Model file for the job. Use its own axes, mm. A direction names the side the tool comes from. Give positions to 0.01 mm unless a question says otherwise; leave off trailing zeros. Order: outer loops, then holes, each group sorted by start corner. A loop starts at its lowest first (then second) coordinate and runs counter-clockwise, first axis right, second up. Notation, with made-up numbers: (63, 22.25) - (95, 22.25) arc R34 cw to (95, 58.25) - close; hole circle Ø1 at (71.25, 61). An arc over 180 degrees is marked (long way). Use CSV: the item, a comma, the result in double quotes. Start each with the question number.
(1) Pull direction Z, two halves, no side cores. Call faces 3 (the flat face through (-25.4, 13, 69)), 4 (the flat face through (-2, 13, 139.7)), 5 (the cylindrical face through (-24.16, 12.88, 9.53)), 6 (the cylindrical face through (-10.907, 1.61, 13.62)): +Z half, -Z half, draft (parallel to the pull), parting line (faces both ways), or undercut.
(2) Band-saw the part on D-D, the plane x = -15.5. Give the cut face in (y, z) (3 decimals), then the cut area to 3 significant figures.
(3) Band-saw the part on A-A, the plane y = 19.25. Give the cut face in (x, z) (3 decimals), then the cut area to 3 significant figures.
(4) Tool access for faces 1 (the flat face through (-13, 0, 69)), 2 (the flat face through (-22.225, 13, 4)): list every direction of +Z, -Z, +X, -X, +Y, -Y with a clear straight run to the whole face (end or side of a thin tool).
(5) Drop flat-ended pins along their axis: pin 1 Ø12 at (x, y) = (-9, 5) entering from -Z; pin 2 Ø4 at (x, z) = (-20.786, 9.68) entering from -Y (3 decimals). Give the stop position or say it passes through.
(6) Band-saw the part on C-C, the plane x = -9.25. Give the cut face in (y, z) (3 decimals), then the cut area to 3 significant figures.
(7) Probe L1, parallel to X at y = 5, z = 68.5 (3 decimals); L2, parallel to Y at x = -18.5, z = 30.5 (3 decimals); L3, parallel to X at y = 19.5, z = 9.68 (3 decimals). List the from-to ranges inside material, lowest first.
(8) Band-saw the part on B-B, the plane z = 16.5. Give the cut face in (x, y) (3 decimals), then the cut area to 3 significant figures.
Autodesk Inventor part; units mm, degrees
ref_plane "YZ Plane" through (0, 0, 0) normal (1, 0, 0) x (0, 1, 0)
ref_plane "XZ Plane" through (0, 0, 0) normal (0, 1, 0) x (-1, 0, 0)
ref_plane "XY Plane" through (0, 0, 0) normal (0, 0, 1) x (1, 0, 0)
sketch "Sketch1" plane through (0, 0, 0) normal (0, 0, 1) x (1, 0, 0)
  line L0 (0, 0) -> (-25.4, 0)
  line L1 (-25.4, 0) -> (-25.4, 25.4)
  line L2 (-25.4, 25.4) -> (0, 25.4)
  line L3 (0, 25.4) -> (0, 0)
  line L4 (-3.175, 22.225) -> (-22.225, 22.225)
  line L5 (-22.225, 22.225) -> (-22.225, 3.175)
  line L6 (-22.225, 3.175) -> (-3.175, 3.175)
  line L7 (-3.175, 3.175) -> (-3.175, 22.225)
  dimension "d0" = 25.4
  dimension "d1" = 25.4
  dimension "d2" = 3.175
extrude "Extrusion1" add sketch "Sketch1" along normal blind 139.7
sketch "Sketch2" plane through (-25.4, 25.4, 0) normal (0, 1, 0) x (1, 0, 0)
  line L0 (0, 0) -> (25.4, 0)
  line L1 (25.4, 0) -> (25.4, -139.7)
  line L2 (0, 0) -> (25.4, -3.8097)
  dimension "d5" = 8.53
extrude "Extrusion2" cut sketch "Sketch2" against normal blind 127
sketch "Sketch3" plane through (-25.4, 25.4, 139.7) normal (0, 1, 0) x (1, 0, 0)
  circle A0 centre (4.614, 130.02) radius 3.3782
  circle A1 centre (17.1735, 128.136) radius 3.3782
  point P0 (25.4, 139.7)
extrude "Extrusion3" cut sketch "Sketch3" against normal blind 63.5
properties part number "V tube" material "Aluminum 6061"
Answer block:
1,face 3,"draft"
1,face 4,"+Z half"
1,face 5,"undercut"
1,face 6,"undercut"
2,outline,"(0, 1.485) - (3.175, 1.485) - (3.175, 139.7) - (0, 139.7) - close; (22.225, 1.485) - (25.4, 1.485) - (25.4, 139.7) - (22.225, 139.7) - close"
2,area,"878 mm2"
3,outline,"(-25.4, 0) - (-22.225, 0.476) - (-22.225, 6.624) arc R3.378 cw to (-22.225, 12.736) - (-22.225, 139.7) - (-25.4, 139.7) - close; (-3.175, 3.333) - (0, 3.81) - (0, 139.7) - (-3.175, 139.7) - close"
3,area,"866 mm2"
4,face 1,"+Z, -Z, +X, -X, -Y"
4,face 2,"+Z, -Z"
5,pin 1,"stops at z = 1.6"
5,pin 2,"passes through"
6,outline,"(0, 2.422) - (3.175, 2.422) - (3.175, 8.345) - (0, 8.345) - close; (0, 14.783) - (3.175, 14.783) - (3.175, 139.7) - (0, 139.7) - close; (22.225, 2.422) - (25.4, 2.422) - (25.4, 8.345) - (22.225, 8.345) - close; (22.225, 14.783) - (25.4, 14.783) - (25.4, 139.7) - (22.225, 139.7) - close"
6,area,"831 mm2"
7,L1,"x = -25.4 to -22.225, -3.175 to 0"
7,L2,"y = 0 to 3.175, 22.225 to 25.4"
7,L3,"x = -25.4 to -24.164, -3.175 to 0"
8,outline,"(-25.4, 0) - (0, 0) - (0, 25.4) - (-25.4, 25.4) - close; hole (-22.225, 3.175) - (-3.175, 3.175) - (-3.175, 22.225) - (-22.225, 22.225) - close"
8,area,"282 mm2"
